from build123d import *

# Parameters (mm, degrees)
F0_W     = 100
F0_H     = 75
F0_W_2   = 25
F0_H_2   = 71.768835
F0_H_3   = 71.77
F1_DEPTH = 5


with BuildPart() as f1:
    # F0 (on Front) → F1 (new body)
    with BuildSketch(Plane.XZ):
        Polygon((14.091592, 244.709768), (-285.908408, 244.709768), (-285.908408, 129.419536), (-285.908408, 64.709768), (14.091592, 64.709768), (14.091592, 69.656026), align=None)
        with Locations((-211.977881, 167.215428)):
            Rectangle(F0_W, F0_H, mode=Mode.SUBTRACT)
        with Locations((-57.973918, 167.215428)):
            Rectangle(F0_W, F0_H, mode=Mode.SUBTRACT)
        Polygon((14.091592, 64.709768), (-285.908408, 64.709768), (-285.908408, 24.709768), (14.091592, 24.709768), (14.091592, 59.763511), align=None)
        Polygon((14.091592, 24.709768), (-285.908408, 24.709768), (-285.908408, 0), (-285.908408, -205.290232), (-197.684959, -205.290232), (-77.684959, -205.290232), (14.091592, -205.290232), align=None)
        with Locations((-251.720655, -77.47348)):
            Rectangle(F0_W_2, F0_H_2, mode=Mode.SUBTRACT)
        Polygon((-135.837302, -155.290232), (-183.15503, -155.290232), (-183.15503, -25.864778), (-134.315275, -25.864778), (-85.475519, -25.864778), (-85.475519, -155.290232), align=None, mode=Mode.SUBTRACT)
        with Locations((-24.452682, -77.472898)):
            Rectangle(F0_W_2, F0_H_3, mode=Mode.SUBTRACT)
    extrude(amount=F1_DEPTH)


solid = f1.part
The model under review builds one solid part; all positions refer to its coordinate system, in mm. Round coordinates to 2 decimals unless told otherwise and drop trailing zeros. Order: outer loops, then holes, each group sorted by start corner. A loop starts at its lowest first (then second) coordinate and runs counter-clockwise, first axis right, second up. Notation, with made-up numbers: (55, -27.5) -> (93, -27.5) arc R9 ccw to (93, -10.5) -> close; hole circle Ø10 at (-18, -16.75). An arc over 180 degrees is marked (long way). Write item = value, one per line. Start each with the question number.
Item 1: For line 1 along Z through (x, y) = (-168.5, -2.5); line 2 along X through (y, z) = (-1.5, 184); line 3 along Z through (x, y) = (-220, -4.1), list the stretches that pass through material, from the lowest coordinate up.
Item 2: Consider section B-B on x = -100.5. Write out the cut boundary in (y, z).
Item 3: Consider section D-D on z = 155.5. Write out the cut boundary in (x, y), plus the area to 3 significant figures.
Item 4: Consider section C-C on y = -3.35. Write out the cut boundary in (x, z), plus the area to 3 significant figures.
Item 5: Consider section A-A on z = -119. Write out the cut boundary in (x, y).
Conclusion:
q1.line_1 = -205.29 to -155.29, -25.86 to 129.72, 204.72 to 244.71
q1.line_2 = -285.91 to -261.98, -161.98 to -107.97, -7.97 to 14.09
q1.line_3 = -205.29 to 129.72, 204.72 to 244.71
q2.outline = (-5, -205.29) -> (0, -205.29) -> (0, -155.29) -> (-5, -155.29) -> close; (-5, -25.86) -> (0, -25.86) -> (0, 129.72) -> (-5, 129.72) -> close; (-5, 204.72) -> (0, 204.72) -> (0, 244.71) -> (-5, 244.71) -> close
q3.outline = (-285.91, -5) -> (-261.98, -5) -> (-261.98, 0) -> (-285.91, 0) -> close; (-161.98, -5) -> (-107.97, -5) -> (-107.97, 0) -> (-161.98, 0) -> close; (-7.97, -5) -> (14.09, -5) -> (14.09, 0) -> (-7.97, 0) -> close
q3.area = 500 mm2
q4.outline = (-285.91, -205.29) -> (14.09, -205.29) -> (14.09, 244.71) -> (-285.91, 244.71) -> close; hole (-264.22, -113.36) -> (-239.22, -113.36) -> (-239.22, -41.59) -> (-264.22, -41.59) -> close; hole (-261.98, 129.72) -> (-161.98, 129.72) -> (-161.98, 204.72) -> (-261.98, 204.72) -> close; hole (-183.16, -155.29) -> (-85.48, -155.29) -> (-85.48, -25.86) -> (-183.16, -25.86) -> close; hole (-107.97, 129.72) -> (-7.97, 129.72) -> (-7.97, 204.72) -> (-107.97, 204.72) -> close; hole (-36.95, -113.36) -> (-11.95, -113.36) -> (-11.95, -41.59) -> (-36.95, -41.59) -> close
q4.area = 104,000 mm2
q5.outline = (-285.91, -5) -> (-183.16, -5) -> (-183.16, 0) -> (-285.91, 0) -> close; (-85.48, -5) -> (14.09, -5) -> (14.09, 0) -> (-85.48, 0) -> close
